The listing builds one solid part. Answer for the finished solid, in the listing's coordinates (mm). A direction names the side the tool comes from. Round coordinates to 2 decimals unless told otherwise and drop trailing zeros. Write each loop counter-clockwise with the first axis right and the second up, starting at its lowest first coordinate (ties: lowest second). Pieces come first, ordered by that corner, then holes.
Item 1: Find section A-A on z = -38.5. Give the vertices of the cut face in (x, y), then the cut area to 3 significant figures.
Item 2: Find the intervals of material crossed by probe 1 along X at (y, z) = (-3.4, -84); probe 2 along Z at (x, y) = (57.5, -2.8); probe 3 along Z at (x, y) = (126.5, -1.5), in increasing order.
Item 3: A tool of negligible diameter and unlimited length cuts with its end or side. For faces 4 (the face through (65.13, -1.97, -49.36)), 5 (the face through (6.271, -2, -55)), from which of +Z, -Z, +X, -X, +Y, -Y can it reach the whole face along a straight path? Write none if from no direction.
Item 4: Find section B-B on x = 93. Give the vertices of the cut face in (y, z), then the cut area to 3 significant figures.
Item 5: For a pull along X with two mould halves and no side action, classify faces 1 (the face through (133.264, -2.028, -13.417)), 2 (the face through (71, -2, -10.565)), 3 (the face through (77.47, -1.97, -49.42)) as +X half, -X half, draft (parallel to the pull), parting line (faces both ways), or undercut.
Item 6: Find section C-C on y = -0.75. Give the number of separate pieces and of enclosed holes in the cut face, then the cut area to 3 significant figures.
```python
from build123d import *

# Parameters (mm, degrees)
SKETCH2_W           = 130
SKETCH2_H           = 90
BOSS_EXTRUDE1_DEPTH = 4
SKETCH3_R           = 1.5
CUT_EXTRUDE1_DEPTH  = 10
SKETCH4_R           = 1.6
CUT_EXTRUDE2_DEPTH  = 10
FILLET1_R           = 10
CUT_EXTRUDE3_DEPTH  = 10


with BuildPart() as part:
    # Sketch2 → Boss-Extrude1 (new body)
    with BuildSketch(Plane(origin=(0, 0, 0), x_dir=(1, 0, 0), z_dir=(0, 1, 0))):
        with Locations((71.271186441, 55.564971751)):
            Rectangle(SKETCH2_W, SKETCH2_H)
    extrude(amount=-BOSS_EXTRUDE1_DEPTH)

    # Sketch3 → Cut-Extrude1 (cut)
    with BuildSketch(Plane(origin=(0, 0, 0), x_dir=(1, 0, 0), z_dir=(0, 1, 0))):
        with Locations(Location((126.271186441, 63.564971751, 0), (0, 0, 270))):
            Circle(SKETCH3_R)
        with Locations(Location((126.271186441, 47.564971751, 0), (0, 0, 270))):
            Circle(SKETCH3_R)
        with Locations(Location((112.271186441, 47.564971751, 0), (0, 0, 270))):
            Circle(SKETCH3_R)
        with Locations(Location((112.271186441, 63.564971751, 0), (0, 0, 270))):
            Circle(SKETCH3_R)
        with Locations(Location((16.271186441, 47.564971751, 0), (0, 0, 90))):
            Circle(SKETCH3_R)
        with Locations(Location((30.271186441, 47.564971751, 0), (0, 0, 90))):
            Circle(SKETCH3_R)
        with Locations(Location((16.271186441, 63.564971751, 0), (0, 0, 90))):
            Circle(SKETCH3_R)
        with Locations(Location((30.271186441, 63.564971751, 0), (0, 0, 90))):
            Circle(SKETCH3_R)
    extrude(amount=-CUT_EXTRUDE1_DEPTH, mode=Mode.SUBTRACT)

    # Sketch4 → Cut-Extrude2 (cut)
    with BuildSketch(Plane(origin=(0, 0, 0), x_dir=(1, 0, 0), z_dir=(0, 1, 0))):
        with Locations(Location((16.271186441, 20.564971751, 0), (0, 0, 270))):
            Circle(SKETCH4_R)
        with Locations(Location((30.271186441, 20.564971751, 0), (0, 0, 270))):
            Circle(SKETCH4_R)
        with Locations(Location((30.271186441, 90.564971751, 0), (0, 0, 90))):
            Circle(SKETCH4_R)
        with Locations(Location((16.271186441, 90.564971751, 0), (0, 0, 90))):
            Circle(SKETCH4_R)
        with Locations(Location((112.271186441, 20.564971751, 0), (0, 0, 90))):
            Circle(SKETCH4_R)
        with Locations(Location((126.271186441, 20.564971751, 0), (0, 0, 90))):
            Circle(SKETCH4_R)
        with Locations(Location((126.271186441, 90.564971751, 0), (0, 0, 270))):
            Circle(SKETCH4_R)
        with Locations(Location((112.271186441, 90.564971751, 0), (0, 0, 270))):
            Circle(SKETCH4_R)
    extrude(amount=-CUT_EXTRUDE2_DEPTH, mode=Mode.SUBTRACT)

    # Fillet1
    fillet1_edges = [part.edges().sort_by_distance(p)[0] for p in [
        (6.271186441, -2, -100.564971751),
        (136.271186441, -2, -100.564971751),
        (136.271186441, -2, -10.564971751),
        (6.271186441, -2, -10.564971751),
    ]]
    fillet(fillet1_edges, radius=FILLET1_R)

    # Sketch5 → Cut-Extrude3 (cut)
    with BuildSketch(Plane(origin=(0, 0, 0), x_dir=(1, 0, 0), z_dir=(0, 1, 0))):
        with BuildLine():
            Line((76.271186441, 89.564971751), (76.271186441, 64.564971751))
            ThreePointArc((76.271186441, 64.564971751), (77.442759316, 61.736544627), (80.271186441, 60.564971751))
            Line((80.271186441, 60.564971751), (98.271186441, 60.564971751))
            ThreePointArc((98.271186441, 60.564971751), (101.099613565, 61.736544627), (102.271186441, 64.564971751))
            Line((102.271186441, 64.564971751), (102.271186441, 89.564971751))
            ThreePointArc((102.271186441, 89.564971751), (101.099613565, 92.393398876), (98.271186441, 93.564971751))
            Line((98.271186441, 93.564971751), (80.271186441, 93.564971751))
            ThreePointArc((80.271186441, 93.564971751), (77.442759316, 92.393398876), (76.271186441, 89.564971751))
        make_face()
        with BuildLine():
            Line((40.271186441, 89.564971751), (40.271186441, 64.564971751))
            ThreePointArc((40.271186441, 64.564971751), (41.442759316, 61.736544627), (44.271186441, 60.564971751))
            Line((44.271186441, 60.564971751), (62.271186441, 60.564971751))
            ThreePointArc((62.271186441, 60.564971751), (65.099613565, 61.736544627), (66.271186441, 64.564971751))
            Line((66.271186441, 64.564971751), (66.271186441, 89.564971751))
            ThreePointArc((66.271186441, 89.564971751), (65.099613565, 92.393398876), (62.271186441, 93.564971751))
            Line((62.271186441, 93.564971751), (44.271186441, 93.564971751))
            ThreePointArc((44.271186441, 93.564971751), (41.442759316, 92.393398876), (40.271186441, 89.564971751))
        make_face()
        with BuildLine():
            Line((66.271186441, 21.564971751), (66.271186441, 46.564971751))
            ThreePointArc((66.271186441, 46.564971751), (65.099613565, 49.393398876), (62.271186441, 50.564971751))
            Line((62.271186441, 50.564971751), (44.271186441, 50.564971751))
            ThreePointArc((44.271186441, 50.564971751), (41.442759316, 49.393398876), (40.271186441, 46.564971751))
            Line((40.271186441, 46.564971751), (40.271186441, 21.564971751))
            ThreePointArc((40.271186441, 21.564971751), (41.442759316, 18.736544627), (44.271186441, 17.564971751))
            Line((44.271186441, 17.564971751), (62.271186441, 17.564971751))
            ThreePointArc((62.271186441, 17.564971751), (65.099613565, 18.736544627), (66.271186441, 21.564971751))
        make_face()
        with BuildLine():
            Line((102.271186441, 21.564971751), (102.271186441, 46.564971751))
            ThreePointArc((102.271186441, 46.564971751), (101.099613565, 49.393398876), (98.271186441, 50.564971751))
            Line((98.271186441, 50.564971751), (80.271186441, 50.564971751))
            ThreePointArc((80.271186441, 50.564971751), (77.442759316, 49.393398876), (76.271186441, 46.564971751))
            Line((76.271186441, 46.564971751), (76.271186441, 21.564971751))
            ThreePointArc((76.271186441, 21.564971751), (77.442759316, 18.736544627), (80.271186441, 17.564971751))
            Line((80.271186441, 17.564971751), (98.271186441, 17.564971751))
            ThreePointArc((98.271186441, 17.564971751), (101.099613565, 18.736544627), (102.271186441, 21.564971751))
        make_face()
    extrude(amount=-CUT_EXTRUDE3_DEPTH, mode=Mode.SUBTRACT)


solid = part.part
```
Check values:
1. outline: (6.27, -4) - (40.27, -4) - (40.27, 0) - (6.27, 0) - close; (66.27, -4) - (76.27, -4) - (76.27, 0) - (66.27, 0) - close; (102.27, -4) - (136.27, -4) - (136.27, 0) - (102.27, 0) - close
1. area: 312 mm2
2. probe 1: x = 6.27 to 40.27, 66.27 to 76.27, 102.27 to 136.27
2. probe 2: z = -100.56 to -93.56, -60.56 to -50.56, -17.56 to -10.56
2. probe 3: z = -100.56 to -92.15, -88.98 to -65.05, -62.08 to -49.05, -46.08 to -22.15, -18.98 to -10.57
3. face 4: +Y, -Y
3. face 5: +Z, -Z, -X, +Y, -Y
4. outline: (-4, -100.56) - (0, -100.56) - (0, -93.56) - (-4, -93.56) - close; (-4, -60.56) - (0, -60.56) - (0, -50.56) - (-4, -50.56) - close; (-4, -17.56) - (0, -17.56) - (0, -10.56) - (-4, -10.56) - close
4. area: 96.0 mm2
5. face 1: +X half
5. face 2: draft
5. face 3: undercut
6. separate pieces: 1
6. enclosed holes: 20
6. area: 8,120 mm2
